Can you work these out from the drawing? Everything is in mm from the part's minimum corner. A direction names the side the tool comes from. Round coordinates to 2 decimals unless told otherwise and drop trailing zeros. Order: outer loops, then holes, each group sorted by start corner. A loop starts at its lowest first (then second) coordinate and runs counter-clockwise, first axis right, second up. Notation, with made-up numbers: (66.5, 72.5) -> (88.5, 72.5) arc R31 ccw to (88.5, 111.5) -> close; hole circle Ø5 at (3, -24). An arc over 180 degrees is marked (long way). Use a Markdown table: item, result. Add a question column.
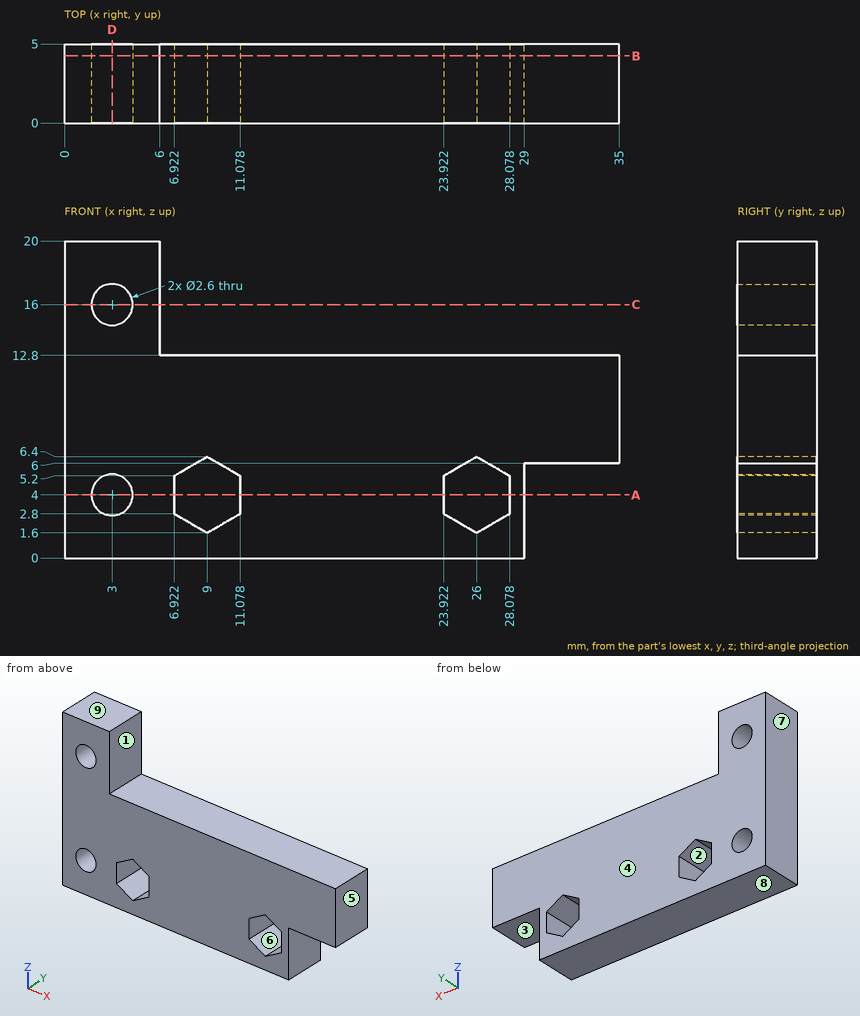
(1) I want a section at D-D on x = 3. List the corners of the cut face in (y, z) for me.
(2) I want a section at B-B on y = 4.25. List the corners of the cut face in (x, z) for me.
(3) On a 3-axis mill with a long thin cutter (end or side, diameter ignored), from which of +Z, -Z, +X, -X, +Y, -Y can I reach the whole of each face in a straight line? I mean the marked faces 1, 2, 3, 4 and 5. Say none if no direction works.
(4) Please list where these lines run through material, in increasing order: probe 1 along Z at (x, y) = (3, 1.15); probe 2 along Z at (x, y) = (2.5, 1.2); probe 3 along X at (y, z) = (1.45, 16). Write a range as from..to.
(5) I want a section at C-C on z = 16. List the corners of the cut face in (x, y) for me.
(6) If we mould it in two halves opening along Z, with no side actions, what happens to the marked faces 6, 7, 8 and 9? For each: pulls with the +Z half, pulls with the -Z half, needs draft (parallel to the pull), parting line crosses it, or undercut.
(7) I'm going to push flat-ended pins straight in: P1, Ø1.5, axis at y = 2, z = 16, coming from the +X side; P2, Ø2.5, axis at x = 17, y = 2.5, coming from the +Z side; P3, Ø1.9, axis at y = 2, z = 4, coming from the +X side; P4, Ø2, axis at x = 3, z = 16, coming from the +Y side. Where does each tip first touch, or does it pass through?
(8) I want a section at A-A on z = 4. List the corners of the cut face in (x, y) for me.
Output:
| question | item | result |
|---|---|---|
| 1 | outline | (0, 0) -> (5, 0) -> (5, 2.7) -> (0, 2.7) -> close; (0, 5.3) -> (5, 5.3) -> (5, 14.7) -> (0, 14.7) -> close; (0, 17.3) -> (5, 17.3) -> (5, 20) -> (0, 20) -> close |
| 2 | outline | (0, 0) -> (29, 0) -> (29, 6) -> (35, 6) -> (35, 12.8) -> (6, 12.8) -> (6, 20) -> (0, 20) -> close; hole circle Ø2.6 at (3, 4); hole circle Ø2.6 at (3, 16); hole (6.92, 2.8) -> (9, 1.6) -> (11.08, 2.8) -> (11.08, 5.2) -> (9, 6.4) -> (6.92, 5.2) -> close; hole (23.92, 2.8) -> (26, 1.6) -> (28.08, 2.8) -> (28.08, 5.2) -> (26, 6.4) -> (23.92, 5.2) -> close |
| 3 | face 1 | +Z, +X, +Y, -Y |
| 3 | face 2 | +Y, -Y |
| 3 | face 3 | -Z, +X, +Y, -Y |
| 3 | face 4 | +Z, -Z, +X, -X, +Y |
| 3 | face 5 | +Z, -Z, +X, +Y, -Y |
| 4 | probe 1 | 0..2.7, 5.3..14.7, 17.3..20 |
| 4 | probe 2 | 0..2.8, 5.2..14.8, 17.2..20 |
| 4 | probe 3 | 0..1.7, 4.3..6 |
| 5 | outline | (0, 0) -> (1.7, 0) -> (1.7, 5) -> (0, 5) -> close; (4.3, 0) -> (6, 0) -> (6, 5) -> (4.3, 5) -> close |
| 6 | face 6 | undercut |
| 6 | face 7 | needs draft |
| 6 | face 8 | pulls with the -Z half |
| 6 | face 9 | pulls with the +Z half |
| 7 | P1 | x = 6 |
| 7 | P2 | z = 12.8 |
| 7 | P3 | x = 29 |
| 7 | P4 | through |
| 8 | outline | (0, 0) -> (1.7, 0) -> (1.7, 5) -> (0, 5) -> close; (4.3, 0) -> (6.92, 0) -> (6.92, 5) -> (4.3, 5) -> close; (11.08, 0) -> (23.92, 0) -> (23.92, 5) -> (11.08, 5) -> close; (28.08, 0) -> (29, 0) -> (29, 5) -> (28.08, 5) -> close |
